Part model, mm, in its own coordinate system. Face numbers are marked on the shaded views. Round coordinates to 2 decimals unless told otherwise and drop trailing zeros. Loops run counter-clockwise (first coordinate to the right, second up) from the corner with the lowest first, then second, coordinate; pieces in that order, holes last. Notation, with made-up numbers: M 9,17.25 L 21,17.25 A9 ccw 21,30.25 Z; hole C -22,23.5 d3. An arc over 180 degrees is marked long. Put each result on its own line as item: value. Start each with the question number.
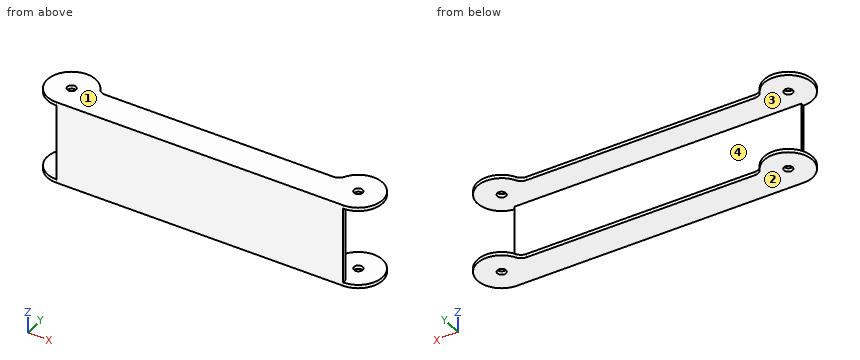
```python
from build123d import *

# Parameters (mm, degrees)
SKETCH2_W                      = 195
SKETCH2_H                      = 48
BOSS_EXTRUDE1_DEPTH            = 14
SHELL1_T                       = -2
SKETCH3_R                      = 2.5
CUT_EXTRUDE1_DEPTH             = 110.573035004
CUT_EXTRUDE2_REACH             = 196.99
SKETCH4_W                      = 44
SKETCH4_H                      = 26
CUT_EXTRUDE2_DIRECTION_2_REACH = 196.99
CUT_EXTRUDE3_DEPTH             = 102.381704464
CUT_EXTRUDE3_DEPTH_BACK        = 102.381704464
CUT_EXTRUDE4_REACH             = 105.307
SKETCH7_W                      = 7.211102551
SKETCH7_H                      = 44
FILLET1_R                      = 5


with BuildPart() as part:
    # Sketch2 → Boss-Extrude1 (new, symmetric)
    with BuildSketch(Plane(origin=(0, 0, 0), x_dir=(1, 0, 0), z_dir=(0, 1, 0))):
        Rectangle(SKETCH2_W, SKETCH2_H)
    extrude(amount=BOSS_EXTRUDE1_DEPTH, both=True)

    # Shell1
    shell1_openings = [part.faces().sort_by_distance(p)[0] for p in [
        (0, 14, 0),
    ]]
    offset(amount=SHELL1_T, openings=shell1_openings, kind=Kind.INTERSECTION)

    # Sketch3 → Cut-Extrude1 (cut, through all)
    with BuildSketch(Plane.XY.offset(24)):
        with Locations((-82.5, 0)):
            Circle(SKETCH3_R)
        with Locations((82.5, 0)):
            Circle(SKETCH3_R)
    extrude(amount=-CUT_EXTRUDE1_DEPTH, mode=Mode.SUBTRACT)

    # Sketch4 → Cut-Extrude2 (cut, up to next)
    with BuildSketch(Plane(origin=(-95.5, 0, 0), x_dir=(0, 0, -1), z_dir=(1, 0, 0)), mode=Mode.PRIVATE) as cut_extrude2_sk1:
        with Locations((0, 1)):
            Rectangle(SKETCH4_W, SKETCH4_H)
    cut_extrude2_tool1 = extrude(cut_extrude2_sk1.sketch, amount=-CUT_EXTRUDE2_REACH, mode=Mode.PRIVATE) & part.part
    add(cut_extrude2_tool1.solids().sort_by_distance((-95.5, 1, 0))[0], mode=Mode.SUBTRACT)

    # Sketch4 → Cut-Extrude2 direction 2 (cut, up to next)
    with BuildSketch(Plane(origin=(-95.5, 0, 0), x_dir=(0, 0, -1), z_dir=(1, 0, 0)), mode=Mode.PRIVATE) as cut_extrude2_direction_2_sk1:
        with Locations((0, 1)):
            Rectangle(SKETCH4_W, SKETCH4_H)
    cut_extrude2_direction_2_tool1 = extrude(cut_extrude2_direction_2_sk1.sketch, amount=CUT_EXTRUDE2_DIRECTION_2_REACH, mode=Mode.PRIVATE) & part.part
    add(cut_extrude2_direction_2_tool1.solids().sort_by_distance((-95.5, 1, 0))[0], mode=Mode.SUBTRACT)

    # Sketch6 → Cut-Extrude3 (cut, two sides: drawn at the far end of the back side and taken through both)
    with BuildSketch(Plane.XY.offset(-CUT_EXTRUDE3_DEPTH_BACK)):
        with BuildLine():
            Line((-69.083592135, 4), (69.083592135, 4))
            ThreePointArc((69.083592135, 4), (93.72497216, 8.366600265), (82.5, -14))
            Line((82.5, -14), (97.5, -14))
            Line((97.5, -14), (97.5, 24))
            Line((97.5, 24), (-97.5, 24))
            Line((-97.5, 24), (-97.5, -14))
            Line((-97.5, -14), (-82.5, -14))
            ThreePointArc((-82.5, -14), (-93.72497216, 8.366600265), (-69.083592135, 4))
        make_face()
    extrude(amount=CUT_EXTRUDE3_DEPTH + CUT_EXTRUDE3_DEPTH_BACK, mode=Mode.SUBTRACT)

    # Sketch7 → Cut-Extrude4 (cut, up to next)
    with BuildSketch(Plane.XZ.offset(14), mode=Mode.PRIVATE) as cut_extrude4_sk1:
        with Locations((86.105551276, 0)):
            Rectangle(SKETCH7_W, SKETCH7_H)
    cut_extrude4_tool1 = extrude(cut_extrude4_sk1.sketch, amount=-CUT_EXTRUDE4_REACH, mode=Mode.PRIVATE) & part.part
    # Sketch7 → Cut-Extrude4 (cut, up to next)
    with BuildSketch(Plane.XZ.offset(14), mode=Mode.PRIVATE) as cut_extrude4_sk2:
        with Locations((-86.105551276, 0)):
            Rectangle(SKETCH7_W, SKETCH7_H)
    cut_extrude4_tool2 = extrude(cut_extrude4_sk2.sketch, amount=-CUT_EXTRUDE4_REACH, mode=Mode.PRIVATE) & part.part
    add(cut_extrude4_tool1.solids().sort_by_distance((86.105551, -14, 0))[0], mode=Mode.SUBTRACT)
    add(cut_extrude4_tool2.solids().sort_by_distance((-86.105551, -14, 0))[0], mode=Mode.SUBTRACT)

    # Fillet1
    fillet1_edges = [part.edges().sort_by_distance(p)[0] for p in [
        (69.083592135, 4, -23),
        (-69.083592135, 4, 23),
        (-69.083592135, 4, -23),
        (69.083592135, 4, 23),
    ]]
    fillet(fillet1_edges, radius=FILLET1_R)


solid = part.part
```
1. Cut at B-B, the plane x = 61. Give the cut face in (y, z), and give its area (3 significant figures).
2. Wall check: L1, parallel to Z at x = 21, y = -5.5; L2, parallel to Y at x = 82.5, z = -22.55; L3, parallel to Y at x = -8, z = -20.5. Give the ranges that are in metal, low to high.
3. Cut at D-D, the plane z = -14. Give the cut face in (x, y).
4. Cut at A-A, the plane y = 0. Give the cut face in (x, z).
5. Cut at C-C, the plane y = 9.25. Give the cut face in (x, z), and give its area (3 significant figures).
6. Drop flat-ended pins along their axis: pin 1 (4 mm diameter, centred on x = -82.5, y = 0, fed in from -Z); pin 2 (2 mm diameter, centred on y = -12.5, z = 7, fed in from +X); pin 3 (2 mm diameter, centred on y = -12.5, z = -7, fed in from -X); pin 4 (13 mm diameter, centred on x = -2, z = -3, fed in from +Y). Give the stop position or say it passes through.
7. Mould opens along Z. For the marked faces 1, 2, 3 and 4 say: released by +Z, released by -Z, zero draft, split by the parting line, or undercut.
Results list:
1. outline: M -14,-24 L 4,-24 L 4,-22 L -12,-22 L -12,22 L 4,22 L 4,24 L -14,24 Z
1. area: 160 mm^2
2. L1: z = -24 to -22, 22 to 24
2. L2: y = -14 to -2.5, 2.5 to 14
2. L3: y = -14 to -12
3. outline: M -82.5,-14 L 82.5,-14 L 82.5,-12 L -82.5,-12 Z
4. outline: M -96.5,-24 L -85,-24 L -85,-22 L -96.5,-22 Z; M -96.5,22 L -85,22 L -85,24 L -96.5,24 Z; M -80,-24 L 80,-24 L 80,-22 L -80,-22 Z; M -80,22 L 80,22 L 80,24 L -80,24 Z; M 85,-24 L 96.5,-24 L 96.5,-22 L 85,-22 Z; M 85,22 L 96.5,22 L 96.5,24 L 85,24 Z
5. outline: M -93.01,-24 L -71.99,-24 L -71.99,-22 L -93.01,-22 Z; M -93.01,22 L -71.99,22 L -71.99,24 L -93.01,24 Z; M 71.99,-24 L 93.01,-24 L 93.01,-22 L 71.99,-22 Z; M 71.99,22 L 93.01,22 L 93.01,24 L 71.99,24 Z
5. area: 168 mm^2
6. pin 1: passes through
6. pin 2: stops at x = 82.5
6. pin 3: stops at x = -82.5
6. pin 4: stops at y = -12
7. face 1: released by +Z
7. face 2: released by -Z
7. face 3: undercut
7. face 4: undercut
